The listing builds one solid part. Answer for the finished solid, in the listing's coordinates (mm). A direction names the side the tool comes from. Give positions to 0.01 mm unless a question says otherwise; leave off trailing zeros. Write each loop counter-clockwise with the first axis right and the second up, starting at its lowest first coordinate (ties: lowest second). Pieces come first, ordered by that corner, then holes. Notation, with made-up numbers: (32, 67.5) - (75, 67.5) arc R6 cw to (75, 72.5) - close; hole circle Ø10 at (-4, -4). An arc over 180 degrees is marked (long way). Write each question's results on one line, items separated by ' | '. Start each with the question number.
Q1. Section B-B (z = 5) is taken. Determine the outline of the cut face in (x, y), plus the area to 3 significant figures.
Q2. Find the intervals of material crossed by probe 1 along Y at (x, z) = (-11.7, 5.6); probe 2 along X at (y, z) = (-1.25, 4.75); probe 3 along X at (y, z) = (2.5, 6.2), in increasing order.
Q3. For a pull along Y with two mould halves and no side action, classify faces 1 (the face through (-11, -7.5, 6)), 2 (the face through (-7.7, -1, 6)), 3 (the face through (-7, 6, 8)) as pulls with the +Y half, pulls with the -Y half, needs draft (parallel to the pull), parting line crosses it, or undercut.
Q4. Flat-ended cylindrical pins translate along their axes: pin 1 Ø2 at (y, z) = (-5, 7) entering from +X; pin 2 Ø0.7 at (x, y) = (-9, 4.5) entering from -Z; pin 3 Ø1.5 at (x, z) = (-4, 5.5) entering from -Y; pin 4 Ø1.1 at (x, z) = (-6.5, 5.5) entering from -Y. Find the tip coordinate at first contact, or state that the pin passes through.
Q5. For faces 4 (the face through (-9, 5, 4.466)), 5 (the face through (-7, -4.5, 6)), 6 (the face through (-12.4, 0.64, 6.23)), determine the directions among +Z, -Z, +X, -X, +Y, -Y from which every point of the face is accessible in a straight line to the end or side of a thin tool.
Q6. Section C-C (x = -6) is taken. Determine the outline of the cut face in (y, z).
Q7. Section A-A (y = 0) is taken. Determine the outline of the cut face in (x, z), plus the area to 3 significant figures.
Q8. Section D-D (x = -16.7) is taken. Determine the outline of the cut face in (y, z), plus the area to 3 significant figures.
```python
from build123d import *

# Parameters (mm, degrees)
BOSS_EXTRUDE1_DEPTH      = 2
BOSS_EXTRUDE2_DEPTH      = 6
SKETCH24_R               = 3.9
BOSS_EXTRUDE5_DEPTH      = 2.3
SKETCH30_W               = 2.408612022
SKETCH30_H               = 1.324178481
CUT_EXTRUDE12_DEPTH      = 8
CUT_EXTRUDE11_DEPTH      = 5.3
FILLET1_R                = 1.5
SKETCH34_R               = 0.75
CUT_EXTRUDE13_DEPTH      = 8
SKETCH35_R               = 0.75
CUT_EXTRUDE14_DEPTH      = 3
CUT_EXTRUDE14_DEPTH_BACK = 8
SKETCH36_R               = 0.95
CUT_EXTRUDE15_DEPTH      = 8
SKETCH37_R               = 2
CUT_EXTRUDE16_DEPTH      = 2.5
SKETCH38_W               = 3
SKETCH38_H               = 1.25
CUT_EXTRUDE17_DEPTH      = 3.6


with BuildPart() as part:
    # Sketch2 → Boss-Extrude1 (new body)
    with BuildSketch(Plane.XY):
        with BuildLine():
            Line((-2.5, 7.5), (-16.7, 7.5))
            Line((-16.7, 7.5), (-20.7, 3.793442666))
            Line((-20.7, 3.793442666), (-20.7, -4.031648778))
            Line((-20.7, -4.031648778), (-15.7, -7.5))
            Line((-15.7, -7.5), (-6.7, -7.5))
            Line((-6.7, -7.5), (-4.2, -5.6))
            ThreePointArc((-4.2, -5.6), (3.130495168, -6.260990337), (7, 0))
            ThreePointArc((7, 0), (4.949747468, 4.949747468), (0, 7))
            Line((0, 7), (0, 7.5))
            Line((0, 7.5), (-2.5, 7.5))
        make_face()
    extrude(amount=BOSS_EXTRUDE1_DEPTH)

    # Sketch4 → Boss-Extrude2 (add)
    with BuildSketch(Plane.XY.offset(2)):
        Polygon((-15.7, -7.5), (-6.7, -7.5), (-6.759079174, -4.5), (-7.7, -4.5), (-7.7, 2), (-5.5, 2), (-5.5, 5.3), (-2.5, 5.3), (-2.5, 7.5), (-16.7, 7.5), (-20.7, 3.793442666), (-20.7, -4.031648778), align=None)
    extrude(amount=BOSS_EXTRUDE2_DEPTH)

    # Sketch24 → Boss-Extrude5 (add)
    with BuildSketch(Plane.XY.offset(2)):
        Circle(SKETCH24_R)
    extrude(amount=BOSS_EXTRUDE5_DEPTH)

    # Sketch30 → Cut-Extrude12 (cut)
    with BuildSketch(Plane(origin=(-5.5, 0, 0), x_dir=(0, 0, -1), z_dir=(1, 0, 0))):
        with Locations((-3.261593395, 4.63791076)):
            Rectangle(SKETCH30_W, SKETCH30_H)
    extrude(amount=-CUT_EXTRUDE12_DEPTH, mode=Mode.SUBTRACT)

    # Sketch28 → Cut-Extrude11 (cut, through all)
    with BuildSketch(Plane.XY.offset(4.3)):
        with BuildLine():
            Line((-1, 1.732050808), (-1, -1.732050808))
            ThreePointArc((-1, -1.732050808), (2, 0), (-1, 1.732050808))
        make_face()
    extrude(amount=-CUT_EXTRUDE11_DEPTH, mode=Mode.SUBTRACT)

    # Fillet1
    fillet1_edges = [part.edges().sort_by_distance(p)[0] for p in [
        (-11.2, -7.5, 0),
        (-8.35, 7.5, 0),
        (-18.7, 5.646721333, 0),
        (-18.2, -5.765824389, 0),
        (-20.7, -0.119103056, 0),
        (-15.7, -7.5, 4),
        (-20.7, -4.031648778, 4),
        (-20.7, 3.793442666, 4),
        (-16.7, 7.5, 4),
    ]]
    fillet(fillet1_edges, radius=FILLET1_R)

    # Sketch34 → Cut-Extrude13 (cut, along a direction that is not the sketch's normal)
    with BuildSketch(Plane.XZ.offset(-2)):
        with Locations((-7, 8)):
            Circle(SKETCH34_R)
    extrude(amount=-CUT_EXTRUDE13_DEPTH, dir=(0.668583388, -0.743637179, 0), mode=Mode.SUBTRACT)

    # Sketch35 → Cut-Extrude14 (cut, two sides, along a direction that is not the sketch's normal)
    with BuildSketch(Plane(origin=(0, -4.5, 0), x_dir=(1, 0, 0), z_dir=(0, 1, 0))) as cut_extrude14_sk:
        with Locations((-8.259079174, -8)):
            Circle(SKETCH35_R)
    extrude(amount=CUT_EXTRUDE14_DEPTH, dir=(0.599919418, 0.80006043, 0), mode=Mode.SUBTRACT)
    extrude(cut_extrude14_sk.sketch, amount=-CUT_EXTRUDE14_DEPTH_BACK, dir=(0.599919418, 0.80006043, 0), mode=Mode.SUBTRACT)

    # Sketch36 → Cut-Extrude15 (cut)
    with BuildSketch(Plane.XY.offset(8)):
        with Locations((-11.7, 0)):
            Circle(SKETCH36_R)
        with Locations((-16.7, 0)):
            Circle(SKETCH36_R)
    extrude(amount=-CUT_EXTRUDE15_DEPTH, mode=Mode.SUBTRACT)

    # Sketch37 → Cut-Extrude16 (cut)
    with BuildSketch(Plane(origin=(0, 0, 0), x_dir=(-1, 0, 0), z_dir=(0, 0, -1))):
        with Locations((11.7, 0)):
            Circle(SKETCH37_R)
        with Locations((16.7, 0)):
            Circle(SKETCH37_R)
    extrude(amount=-CUT_EXTRUDE16_DEPTH, mode=Mode.SUBTRACT)

    # Sketch38 → Cut-Extrude17 (cut)
    with BuildSketch(Plane.XY.offset(8)):
        with Locations((-4, 5.925)):
            Rectangle(SKETCH38_W, SKETCH38_H)
    extrude(amount=-CUT_EXTRUDE17_DEPTH, mode=Mode.SUBTRACT)


with BuildPart() as body_2:
    # Split1: the piece on the far side of the plane
    add(part.part)
    split(bisect_by=Plane.XY.offset(4.4), keep=Keep.BOTTOM)


with BuildPart() as part_1:
    add(part.part)

    # Split1
    split(bisect_by=Plane.XY.offset(4.4), keep=Keep.TOP)


solid = part_1.part
```
Answers below:
1) outline: (-20.7, -3.25) arc R1.5 ccw to (-20.05, -4.48) - (-16.09, -7.23) arc R1.5 ccw to (-15.23, -7.5) - (-6.7, -7.5) - (-6.76, -4.5) - (-7.7, -4.5) - (-7.7, 2) - (-5.5, 2) - (-5.5, 6.55) - (-2.5, 6.55) - (-2.5, 7.5) - (-16.11, 7.5) arc R1.5 ccw to (-17.13, 7.1) - (-20.22, 4.24) arc R1.5 ccw to (-20.7, 3.14) - close; hole circle Ø1.9 at (-16.7, 0); hole circle Ø1.9 at (-11.7, 0) | area: 191 mm2
2) probe 1: y = -7.5 to -0.95, 0.95 to 7.5 | probe 2: x = -20.7 to -7.7 | probe 3: x = -20.7 to -5.5
3) face 1: pulls with the -Y half | face 2: undercut | face 3: needs draft
4) pin 1: stops at x = -6.73 | pin 2: stops at z = 4.47 | pin 3: stops at y = 6.55 | pin 4: stops at y = -7.5
5) face 4: -Z, +X | face 5: +Z, -Z, +X | face 6: +Z, -Z
6) outline: (2, 4.4) - (3.98, 4.4) - (3.98, 4.47) - (5.3, 4.47) - (5.3, 4.4) - (7.5, 4.4) - (7.5, 8) - (2, 8) - close
7) outline: (-20.7, 4.4) - (-17.65, 4.4) - (-17.65, 8) - (-20.7, 8) - close; (-15.75, 4.4) - (-12.65, 4.4) - (-12.65, 8) - (-15.75, 8) - close; (-10.75, 4.4) - (-7.7, 4.4) - (-7.7, 8) - (-10.75, 8) - close | area: 33.1 mm2
8) outline: (-6.81, 4.4) - (-0.95, 4.4) - (-0.95, 8) - (-6.81, 8) - close; (0.95, 4.4) - (7.38, 4.4) - (7.38, 8) - (0.95, 8) - close | area: 44.2 mm2
